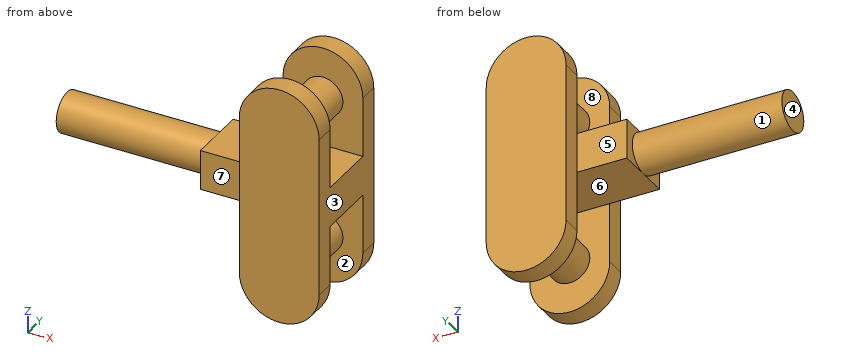
from build123d import *

# Parameters (mm, degrees)
ESQUISSE1_W             = 8
ESQUISSE1_H             = 24
BOSS_EXTRU_1_DEPTH      = 10
ESQUISSE2_W             = 10
ESQUISSE2_H             = 6
ENL_V_MAT_EXTRU_1_DEPTH = 10
ESQUISSE3_R             = 2
BOSS_EXTRU_2_DEPTH      = 6
CONG_1_RADIUS           = 4
CONG_1_LENGTH           = 2
CONG_2_RADIUS           = 4
CONG_2_LENGTH           = 2
CONG_3_RADIUS           = 4
CONG_3_LENGTH           = 2
CONG_4_RADIUS           = 4
CONG_4_LENGTH           = 2
ESQUISSE4_R             = 2
BOSS_EXTRU_3_DEPTH      = 20
ESQUISSE5_W             = 4
ESQUISSE5_H             = 6
BOSS_EXTRU_4_DEPTH      = 5


with BuildPart() as part:
    # Esquisse1 → Boss.-Extru.1 (new body)
    with BuildSketch(Plane(origin=(0, 0, 0), x_dir=(1, 0, 0), z_dir=(0, 1, 0))):
        with Locations((4, 12)):
            Rectangle(ESQUISSE1_W, ESQUISSE1_H)
    extrude(amount=BOSS_EXTRU_1_DEPTH)

    # Esquisse2 → Enlèv. mat.-Extru.1 (cut)
    with BuildSketch(Plane(origin=(8, 0, 0), x_dir=(0, 0, -1), z_dir=(1, 0, 0))):
        with Locations((5, 5)):
            Rectangle(ESQUISSE2_W, ESQUISSE2_H)
        with Locations((19, 5)):
            Rectangle(ESQUISSE2_W, ESQUISSE2_H)
    extrude(amount=-ENL_V_MAT_EXTRU_1_DEPTH, mode=Mode.SUBTRACT)

    # Esquisse3 → Boss.-Extru.2 (add)
    with BuildSketch(Plane(origin=(0, 2, 0), x_dir=(1, 0, 0), z_dir=(0, 1, 0))):
        with Locations(Location((4, 5, 0), (0, 0, 90))):
            Circle(ESQUISSE3_R)
        with Locations(Location((4, 19, 0), (0, 0, 90))):
            Circle(ESQUISSE3_R)
    extrude(amount=BOSS_EXTRU_2_DEPTH)

    # Congé1: full round fillet: the end face becomes a half cylinder, R = half its width
    cong_1_face = Plane((4, 1, -24), x_dir=(0, 1, 0), z_dir=(0, 0, -1))  # on the end face: x along it, z out of the body
    cong_1_slab = cong_1_face.offset(-CONG_1_RADIUS / 2) * Box(CONG_1_LENGTH, 2 * CONG_1_RADIUS, CONG_1_RADIUS, mode=Mode.PRIVATE)  # the body's end, R deep
    cong_1_round = Plane((4, 1, -20), x_dir=(0, 0, -1), z_dir=(0, 1, 0)) * Cylinder(CONG_1_RADIUS, CONG_1_LENGTH, mode=Mode.PRIVATE)  # its axis R under the face
    add(cong_1_slab - cong_1_round, mode=Mode.SUBTRACT)

    # Congé2: full round fillet: the end face becomes a half cylinder, R = half its width
    cong_2_face = Plane((4, 9, -24), x_dir=(0, 1, 0), z_dir=(0, 0, -1))  # on the end face: x along it, z out of the body
    cong_2_slab = cong_2_face.offset(-CONG_2_RADIUS / 2) * Box(CONG_2_LENGTH, 2 * CONG_2_RADIUS, CONG_2_RADIUS, mode=Mode.PRIVATE)  # the body's end, R deep
    cong_2_round = Plane((4, 9, -20), x_dir=(0, 0, -1), z_dir=(0, 1, 0)) * Cylinder(CONG_2_RADIUS, CONG_2_LENGTH, mode=Mode.PRIVATE)  # its axis R under the face
    add(cong_2_slab - cong_2_round, mode=Mode.SUBTRACT)

    # Congé3: full round fillet: the end face becomes a half cylinder, R = half its width
    cong_3_face = Plane((4, 9, 0), x_dir=(0, 1, 0), z_dir=(0, 0, 1))  # on the end face: x along it, z out of the body
    cong_3_slab = cong_3_face.offset(-CONG_3_RADIUS / 2) * Box(CONG_3_LENGTH, 2 * CONG_3_RADIUS, CONG_3_RADIUS, mode=Mode.PRIVATE)  # the body's end, R deep
    cong_3_round = Plane((4, 9, -4), x_dir=(0, 0, 1), z_dir=(0, 1, 0)) * Cylinder(CONG_3_RADIUS, CONG_3_LENGTH, mode=Mode.PRIVATE)  # its axis R under the face
    add(cong_3_slab - cong_3_round, mode=Mode.SUBTRACT)

    # Congé4: full round fillet: the end face becomes a half cylinder, R = half its width
    cong_4_face = Plane((4, 1, 0), x_dir=(0, 1, 0), z_dir=(0, 0, 1))  # on the end face: x along it, z out of the body
    cong_4_slab = cong_4_face.offset(-CONG_4_RADIUS / 2) * Box(CONG_4_LENGTH, 2 * CONG_4_RADIUS, CONG_4_RADIUS, mode=Mode.PRIVATE)  # the body's end, R deep
    cong_4_round = Plane((4, 1, -4), x_dir=(0, 0, 1), z_dir=(0, 1, 0)) * Cylinder(CONG_4_RADIUS, CONG_4_LENGTH, mode=Mode.PRIVATE)  # its axis R under the face
    add(cong_4_slab - cong_4_round, mode=Mode.SUBTRACT)

    # Esquisse4 → Boss.-Extru.3 (add)
    with BuildSketch(Plane.ZY):
        with Locations((-12, 5)):
            Circle(ESQUISSE4_R)
    extrude(amount=BOSS_EXTRU_3_DEPTH)

    # Esquisse5 → Boss.-Extru.4 (add)
    with BuildSketch(Plane.ZY):
        with Locations((-12, 5)):
            Rectangle(ESQUISSE5_W, ESQUISSE5_H)
    extrude(amount=BOSS_EXTRU_4_DEPTH)


solid = part.part
Geometry check sheet. Reference: the model listing, model coordinates, mm. Face numbers are marked on the shaded views. A direction names the side the tool comes from. Round coordinates to 2 decimals unless told otherwise and drop trailing zeros. Loops run counter-clockwise (first coordinate to the right, second up) from the corner with the lowest first, then second, coordinate; pieces in that order, holes last. Notation, with made-up numbers: (39.25, 24) -> (85.25, 24) arc R5 cw to (85.25, 31) -> close; hole circle Ø6 at (25.5, -35.5). An arc over 180 degrees is marked (long way). Answer as a JSON object with one key per item and string values. Group by question number.
Item 1: Cross-section at D-D, the plane x = -10.75. Record the cut outline in (y, z).
Item 2: Set-up check for the marked faces 4, 5, 6, 7 and 8: record each of +Z, -Z, +X, -X, +Y, -Y from which the full face is reachable in a straight line by a thin tool's end or side.
Item 3: Cross-section at A-A, the plane z = -12. Record the cut outline in (x, y).
Item 4: Cross-section at C-C, the plane x = 4. Record the cut outline in (y, z).
Item 5: Thickness scan on line 1 along Y through (x, z) = (5.5, -22.25); line 2 along Y through (x, z) = (-8.5, -12); line 3 along Y through (x, z) = (-4.5, -11.5). Record the ranges inside material, lowest first.
Item 6: Depth check by flat-ended pin: pin 1 Ø3 at (x, z) = (-2, -12) entering from -Y; pin 2 Ø1.8 at (x, y) = (4.5, 4.5) entering from +Z; pin 3 Ø1 at (y, z) = (1, -9) entering from -X. Enter the tip coordinate at first touch or a pass-through.
Item 7: Release check for a two-part mould opening along Z. For the marked faces 1, 2 and 3 record: pulls with the +Z half, pulls with the -Z half, needs draft (parallel to the pull), parting line crosses it, or undercut.
Item 8: Cross-section at B-B, the plane y = 3.5. Record the cut outline in (x, z), plus the area to 3 significant figures.
Determined:
{
 "1": {"outline": "circle Ø4 at (5, -12)"},
 "2": {"face 4": "+Z, -Z, -X, +Y, -Y", "face 5": "+Z, -Z, -X, +Y", "face 6": "+X, -X", "face 7": "+Z, -Z, -X, -Y", "face 8": "none"},
 "3": {"outline": "(-20, 3) -> (-5, 3) -> (-5, 2) -> (0, 2) -> (0, 0) -> (8, 0) -> (8, 10) -> (0, 10) -> (0, 8) -> (-5, 8) -> (-5, 7) -> (-20, 7) -> close"},
 "4": {"outline": "(0, -24) -> (2, -24) -> (2, -21) -> (8, -21) -> (8, -24) -> (10, -24) -> (10, 0) -> (8, 0) -> (8, -3) -> (2, -3) -> (2, 0) -> (0, 0) -> close; hole (2, -17) -> (8, -17) -> (8, -14) -> (2, -14) -> close; hole (2, -10) -> (8, -10) -> (8, -7) -> (2, -7) -> close"},
 "5": {"line 1": "y = 0 to 2, 8 to 10", "line 2": "y = 3 to 7", "line 3": "y = 2 to 8"},
 "6": {"pin 1": "stops at y = 2", "pin 2": "stops at z = -3", "pin 3": "stops at x = 0"},
 "7": {"face 1": "parting line crosses it", "face 2": "undercut", "face 3": "needs draft"},
 "8": {"outline": "(-20, -13.32) -> (-5, -13.32) -> (-5, -14) -> (8, -14) -> (8, -10) -> (-5, -10) -> (-5, -10.68) -> (-20, -10.68) -> close; circle Ø4 at (4, -19); circle Ø4 at (4, -5)", "area": "117 mm²"}
}
